from build123d import *

# Parameters (mm, degrees)
SKETCH_1_W          = 36
SKETCH_1_H          = 24
EXTRUDE_1_DEPTH     = 55
SKETCH_2_R          = 6
CUT_EXTRUDE_1_DEPTH = 36
SKETCH_3_R          = 3.1
CUT_EXTRUDE_2_DEPTH = 6
SKETCH_5_W          = 18
SKETCH_5_H          = 10
EXTRUDE_2_DEPTH     = 36
SKETCH_6_R          = 1.45
CUT_EXTRUDE_3_DEPTH = 5
SKETCH_7_W          = 36
SKETCH_7_H          = 55
EXTRUDE_3_DEPTH     = 3
SKETCH_8_W          = 36
SKETCH_8_H          = 27
CUT_EXTRUDE_4_DEPTH = 3
SKETCH_9_R          = 1.45
CUT_EXTRUDE_5_DEPTH = 1.5


with BuildPart() as part:
    # 草图1 → 凸台-拉伸1 (new body)
    with BuildSketch(Plane(origin=(0, 0, 0), x_dir=(1, 0, 0), z_dir=(0, 1, 0))):
        with Locations((18, 12)):
            Rectangle(SKETCH_1_W, SKETCH_1_H)
    extrude(amount=EXTRUDE_1_DEPTH)

    # 草图2 → 切除-拉伸1 (cut)
    with BuildSketch(Plane.ZY):
        with Locations((-14, 23)):
            Circle(SKETCH_2_R)
    extrude(amount=-CUT_EXTRUDE_1_DEPTH, mode=Mode.SUBTRACT)

    # 草图3 → 切除-拉伸2 (cut)
    with BuildSketch(Plane.XY):
        with Locations((8, 10)):
            Circle(SKETCH_3_R)
        with Locations((28, 10)):
            Circle(SKETCH_3_R)
    extrude(amount=-CUT_EXTRUDE_2_DEPTH, mode=Mode.SUBTRACT)

    # 草图5 → 凸台-拉伸2 (add)
    with BuildSketch(Plane(origin=(36, 0, 0), x_dir=(0, 0, -1), z_dir=(1, 0, 0))):
        with Locations((-9, 50)):
            Rectangle(SKETCH_5_W, SKETCH_5_H)
    extrude(amount=-EXTRUDE_2_DEPTH)

    # 草图6 → 切除-拉伸3 (cut)
    with BuildSketch(Plane(origin=(0, 55, 0), x_dir=(1, 0, 0), z_dir=(0, 1, 0))):
        with Locations(Location((28, -9, 0), (0, 0, 270))):
            Circle(SKETCH_6_R)
        with Locations(Location((8, -9, 0), (0, 0, 270))):
            Circle(SKETCH_6_R)
    extrude(amount=-CUT_EXTRUDE_3_DEPTH, mode=Mode.SUBTRACT)

    # 草图7 → 凸台-拉伸3 (add)
    with BuildSketch(Plane(origin=(0, 0, -24), x_dir=(-1, 0, 0), z_dir=(0, 0, -1))):
        with Locations((-18, 27.5)):
            Rectangle(SKETCH_7_W, SKETCH_7_H)
    extrude(amount=EXTRUDE_3_DEPTH)

    # 草图8 → 切除-拉伸4 (cut)
    with BuildSketch(Plane.XZ):
        with Locations((18, -13.5)):
            Rectangle(SKETCH_8_W, SKETCH_8_H)
    extrude(amount=-CUT_EXTRUDE_4_DEPTH, mode=Mode.SUBTRACT)

    # 草图9 → 切除-拉伸5 (cut)
    with BuildSketch(Plane(origin=(0, 50, 0), x_dir=(1, 0, 0), z_dir=(0, 1, 0))):
        with Locations(Location((8, -9, 0), (0, 0, 270))):
            Circle(SKETCH_9_R)
    extrude(amount=-CUT_EXTRUDE_5_DEPTH, mode=Mode.SUBTRACT)


solid = part.part
Could you check a few things on this model? Use its own coordinates, in mm. A direction names the side the tool comes from. Give positions to 0.01 mm unless a question says otherwise; leave off trailing zeros. Order: outer loops, then holes, each group sorted by start corner. A loop starts at its lowest first (then second) coordinate and runs counter-clockwise, first axis right, second up. Notation, with made-up numbers: (-35, 27) - (10, 27) arc R35 cw to (10, 61) - close; hole circle Ø11 at (-3, 7). An arc over 180 degrees is marked (long way). One line per item, written item: value. Start each with the question number.
1. Imagine slicing it at A-A on y = 23. List the corners of the cut face in (x, z) for me.
2. If I drill on probe 1 along X at (y, z) = (52, 9); probe 2 along Y at (x, z) = (28, -2.5); probe 3 along Z at (x, y) = (16, 34.5), over which ranges is the centre line in solid material (lowest first)?
3. Imagine slicing it at D-D on y = 10. List the corners of the cut face in (x, z) for me.
4. Imagine slicing it at C-C on x = 28. List the corners of the cut face in (y, z) for me.
5. Imagine slicing it at B-B on z = -14. List the corners of the cut face in (x, y) for me.
6. Thinking about a two-plate mould opening in Y: for faces 1 (the face through (18, 55, -4)), 2 (the face through (18, 50, 18)), 3 (the face through (8, 10, -6)), which applies, +Y half, -Y half, draft (parallel to the pull), parting line (faces both ways), or undercut?
7. For faces 4 (the face through (18, 3, -13)), 5 (the face through (18, 24, 0)), 6 (the face through (24.9, 10.1, -3)), 7 (the face through (28, 50, 9)), which set-ups out of +Z, -Z, +X, -X, +Y, -Y let a thin tool reach every point of the face, with its end or its side?
8. For P1, Ø2.5, axis at x = 28.5, z = 9.5, coming from the +Y side; P2, Ø9, axis at x = 21, z = 9.5, coming from the -Y side; P3, Ø3, axis at x = 29.5, y = 11, coming from the +Z side; P4, Ø2.5, axis at x = 8, z = 9, coming from the +Y side, each with a flat end and sliding along its axis, tell me the tip position at first contact or that it passes through.
Values:
1. outline: (0, -27) - (36, -27) - (36, -20) - (0, -20) - close; (0, -8) - (36, -8) - (36, 0) - (0, 0) - close
2. probe 1: 0 to 6.55, 9.45 to 26.55, 29.45 to 36
2. probe 2: 3 to 6.9, 13.1 to 55
2. probe 3: -27 to 0
3. outline: (0, -27) - (36, -27) - (36, 0) - (31.1, 0) - (31.1, -6) - (24.9, -6) - (24.9, 0) - (11.1, 0) - (11.1, -6) - (4.9, -6) - (4.9, 0) - (0, 0) - close
4. outline: (3, -27) - (55, -27) - (55, 7.55) - (50, 7.55) - (50, 10.45) - (55, 10.45) - (55, 18) - (45, 18) - (45, 0) - (13.1, 0) - (13.1, -6) - (6.9, -6) - (6.9, 0) - (3, 0) - close; hole circle Ø12 at (23, -14)
5. outline: (0, 3) - (36, 3) - (36, 17) - (0, 17) - close; (0, 29) - (36, 29) - (36, 55) - (0, 55) - close
6. face 1: +Y half
6. face 2: draft
6. face 3: undercut
7. face 4: +Z, -Z, +X, -X, -Y
7. face 5: +Z, +X, -X, -Y
7. face 6: +Z
7. face 7: +Y
8. P1: y = 55
8. P2: y = 45
8. P3: z = 0
8. P4: y = 48.5
